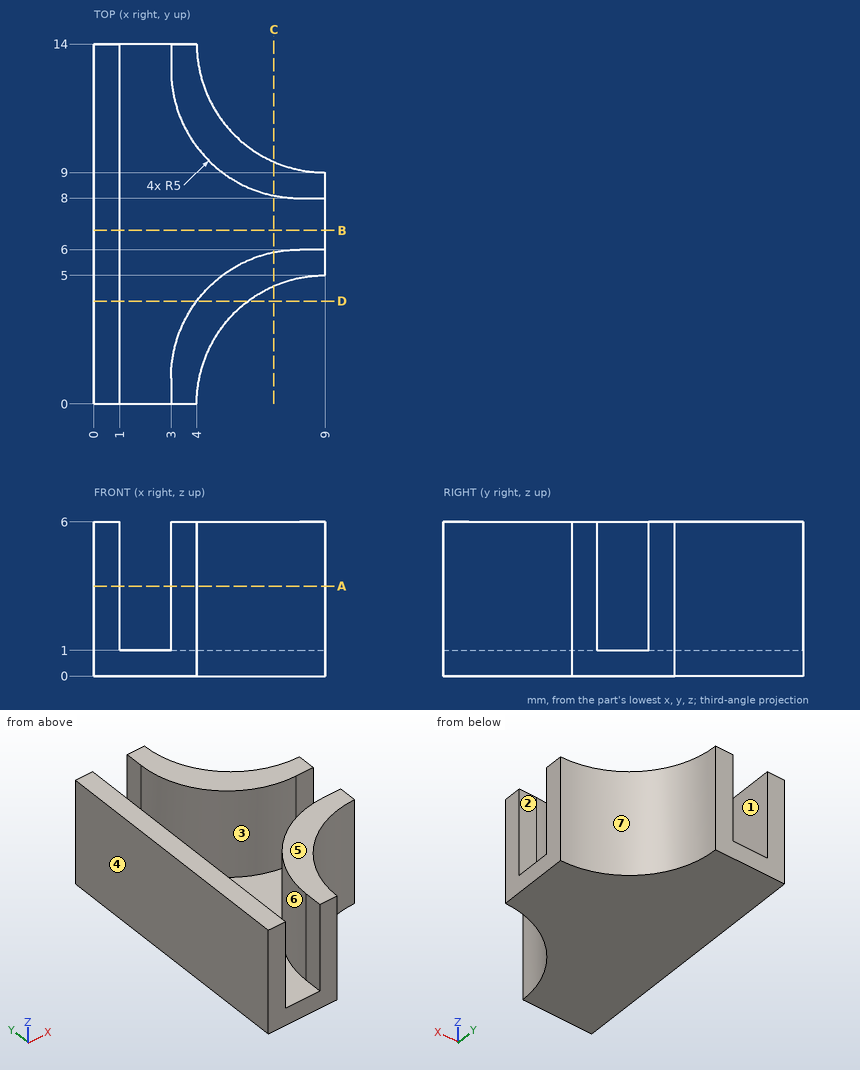
The drawing under review shows one solid part. Ordinate dimensions are in mm from its lowest x, y, z. A direction names the side the tool comes from. Round coordinates to 2 decimals unless told otherwise and drop trailing zeros. Order: outer loops, then holes, each group sorted by start corner. A loop starts at its lowest first (then second) coordinate and runs counter-clockwise, first axis right, second up. Notation, with made-up numbers: (-10, 10.25) -> (48, 10.25) arc R6 ccw to (48, 21.25) -> close; hole circle Ø6 at (-12.5, -40). An arc over 180 degrees is marked (long way). Return JSON: item names as keys, results as strings.
1. Take a section at A-A (z = 3.5). State how many separate pieces and enclosed holes the cut face has, then the cut area to 3 significant figures.
Answer block:
{"separate pieces": "3", "enclosed holes": "0", "area": "36.0 mm²"}
2. For L1, parallel to X at y = 10, z = 4.5; L2, parallel to Y at x = 5, z = 4.7; L3, parallel to Y at x = 6.75, z = 4.45, list the stretches that pass through material, from the lowest coordinate up. Write a range as [from, to].
Answer block:
{"L1": "x = [0, 1], [4, 6]", "L2": "y = [3, 5], [9, 11]", "L3": "y = [4.47, 5.84], [8.16, 9.53]"}
3. Insertion check: P1, Ø1.1, axis at x = 8.5, z = 3.5, coming from the -Y side; P2, Ø1.1, axis at x = 8.5, z = 2.5, coming from the +Y side; P3, Ø1.5, axis at x = 2.5, y = 6, coming from the +Z side. Each pin has a flat end and moves straight along its axis. Give the tip position at first contact, or say it passes through.
Answer block:
{"P1": "stops at y = 4.89", "P2": "stops at y = 9.11", "P3": "stops at z = 1"}
4. For the marked faces 1, 2 and 3, list the 3-axis set-ups (+Z, -Z, +X, -X, +Y, -Y) from which the entire face can be reached by the end or side of a thin tool; tool diameter is ignored.
Answer block:
{"face 1": "+Z, +Y, -Y", "face 2": "+Z, +X", "face 3": "+Z"}
5. The part is to be moulded in two halves that separate along X. For the marked faces 4, 5, 6 and 7, say which applies: +X half, -X half, draft (parallel to the pull), parting line (faces both ways), or undercut.
Answer block:
{"face 4": "-X half", "face 5": "draft", "face 6": "undercut", "face 7": "+X half"}
6. Take a section at D-D (y = 4). Write out the cut boundary in (x, z), then the cut area to 3 significant figures.
Answer block:
{"outline": "(0, 0) -> (6, 0) -> (6, 6) -> (4, 6) -> (4, 1) -> (1, 1) -> (1, 6) -> (0, 6) -> close", "area": "21.0 mm²"}
7. Take a section at B-B (y = 6.75). Write out the cut boundary in (x, z), then the cut area to 3 significant figures.
Answer block:
{"outline": "(0, 0) -> (9, 0) -> (9, 1) -> (1, 1) -> (1, 6) -> (0, 6) -> close", "area": "14.0 mm²"}
8. Take a section at C-C (x = 7). Write out the cut boundary in (y, z).
Answer block:
{"outline": "(4.58, 0) -> (9.42, 0) -> (9.42, 6) -> (8.1, 6) -> (8.1, 1) -> (5.9, 1) -> (5.9, 6) -> (4.58, 6) -> close"}
